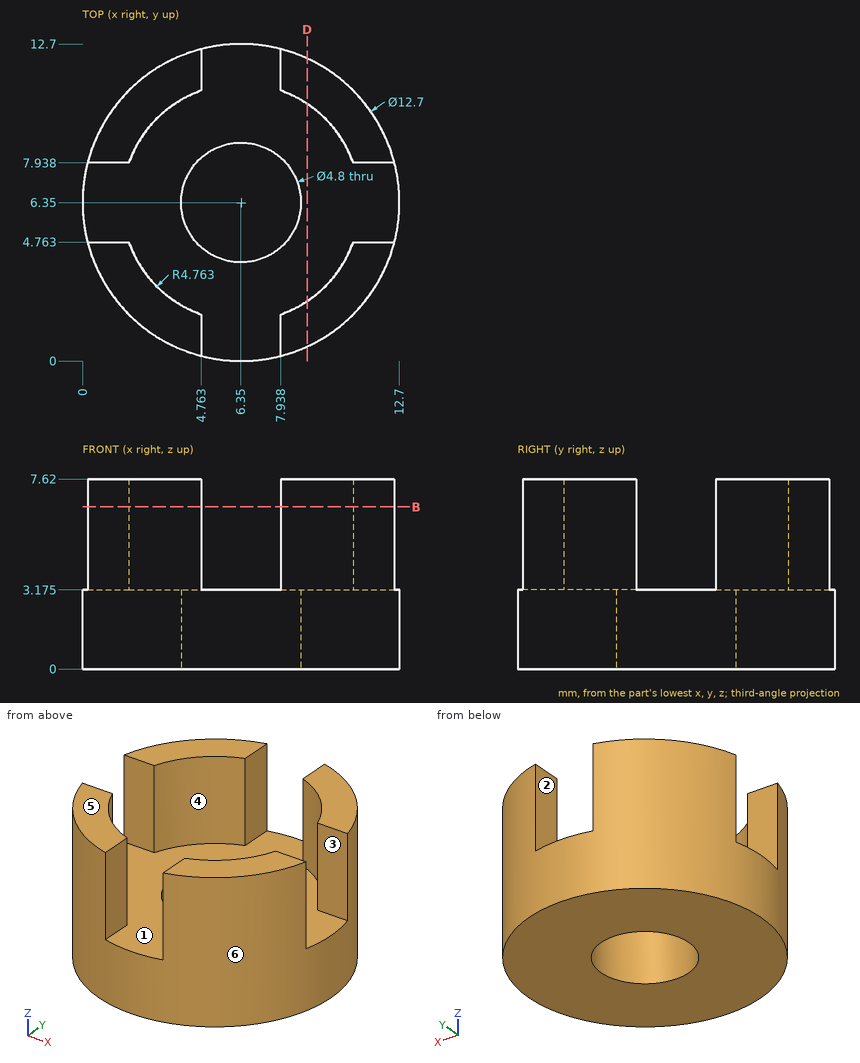
The drawing under review shows one solid part. Ordinate dimensions are in mm from its lowest x, y, z. A direction names the side the tool comes from. Round coordinates to 2 decimals unless told otherwise and drop trailing zeros. Order: outer loops, then holes, each group sorted by start corner. A loop starts at its lowest first (then second) coordinate and runs counter-clockwise, first axis right, second up. Notation, with made-up numbers: (-39.75, 36.5) -> (-18.75, 36.5) arc R5 cw to (-18.75, 45.5) -> close; hole circle Ø2 at (-4.75, 40). An arc over 180 degrees is marked (long way). Return JSON: item names as keys, results as strings.
1. Take a section at D-D (x = 9). Write out the cut boundary in (y, z) (1 decimal).
Answer block:
{"outline": "(0.6, 0) -> (12.1, 0) -> (12.1, 7.6) -> (10.3, 7.6) -> (10.3, 3.2) -> (2.4, 3.2) -> (2.4, 7.6) -> (0.6, 7.6) -> close"}
2. The part is to be moulded in two halves that separate along Y. For the marked faces 4, 5 and 6, say which applies: +Y half, -Y half, draft (parallel to the pull), parting line (faces both ways), or undercut.
Answer block:
{"face 4": "undercut", "face 5": "draft", "face 6": "parting line"}
3. Insertion check: P1, Ø5, axis at x = 5.5, y = 3.5, coming from the +Z side; P2, Ø1.5, axis at x = 8, y = 7, coming from the +Z side (1 decimal); P3, Ø1.3, axis at x = 12, z = 6.5, coming from the +Y side (1 decimal); P4, Ø3, axis at x = 11, z = 1, coming from the +Y side (1 decimal). Each pin has a flat end and moves straight along its axis. Give the tip position at first contact, or say it passes through.
Answer block:
{"P1": "stops at z = 7.62", "P2": "stops at z = 3.2", "P3": "stops at y = 10.3", "P4": "stops at y = 11.9"}
4. For the marked faces 1, 2 and 3, list the 3-axis set-ups (+Z, -Z, +X, -X, +Y, -Y) from which the entire face can be reached by the end or side of a thin tool; tool diameter is ignored.
Answer block:
{"face 1": "+Z", "face 2": "+Z, +Y, -Y", "face 3": "+Z, +X, -X"}
5. For L1, parallel to Y at x = 6.35, z = 2; L2, parallel to Y at x = 1.25, z = 3.75 (1 decimal); L3, parallel to Z at x = 11.75, y = 7.25 (1 decimal), list the stretches that pass through material, from the lowest coordinate up. Write a range as [from, to].
Answer block:
{"L1": "y = [0, 3.95], [8.75, 12.7]", "L2": "y = [2.6, 4.8], [7.9, 10.1]", "L3": "z = [0, 3.2]"}
6. Take a section at B-B (z = 6.5). State how many separate pieces and enclosed holes the cut face has.
Answer block:
{"separate pieces": "4", "enclosed holes": "0"}
